The model under review builds one solid part; all positions refer to its coordinate system, in mm. A direction names the side the tool comes from. Round coordinates to 2 decimals unless told otherwise and drop trailing zeros. Order: outer loops, then holes, each group sorted by start corner. A loop starts at its lowest first (then second) coordinate and runs counter-clockwise, first axis right, second up.
1) Mouldability with a two-part tool opening along Z and no side actions: class faces 3 (the face through (38.1, 2, -3)), 4 (the face through (19, 1, 7.62)), 5 (the face through (34.148, 1.252, 1.164)) as pulls with the +Z half, pulls with the -Z half, needs draft (parallel to the pull), parting line crosses it, or undercut.
2) Consider section A-A (x = 31.75). Give the boundary of the cut face in (y, z).
3) To check wall thickness, follow L1, parallel to Z at x = 6.35, y = 1.75; L2, parallel to Y at x = 22.5, z = 0.75; L3, parallel to Z at x = 11, y = 7.5. State the ranges of each line that lie inside material, in increasing order.
4) Clearance check with flat-ended pins moving along their axes: P1, Ø2.5, axis at x = 27.5, y = 5.5, coming from the +Z side; P2, Ø3, axis at x = 4.5, y = 3.5, coming from the +Z side; P3, Ø7.5, axis at x = 22, z = -2, coming from the +Y side; P4, Ø3, axis at x = 31.75, z = 1.27, coming from the -Y side. State where each tip first meets the part, or that it passes through.
5) Machinability: for faces 1 (the face through (0, 2, -3)), 2 (the face through (19, 2.54, 0)), which of the approach directions +Z, -Z, +X, -X, +Y, -Y give a long, thin tool a straight path to every point of the face, cutting with its end or side? Answer none if there is none.
6) Consider section B-B (z = 1.27). Give the boundary of the cut face in (x, y).
7) Consider section C-C (y = 6.35). Give the boundary of the cut face in (x, z).
8) Consider section D-D (x = 3). Give the boundary of the cut face in (y, z).
from build123d import *

# Parameters (mm, degrees)
SKETCH2_W               = 10.16
SKETCH2_H               = 10.16
BOSS_EXTRUDE1_DEPTH     = 38.1
CUT_EXTRUDE1_DEPTH      = 41.719297636
CUT_EXTRUDE1_DEPTH_BACK = 38.1
SKETCH3_W               = 7.62
SKETCH3_H               = 7.62
M4_CLEARANCE_HOLE2_D    = 4.8
SKETCH13_W              = 38.1
SKETCH13_H              = 2.54
BOSS_EXTRUDE2_DEPTH     = 7.62
M4_CLEARANCE_HOLE3_D    = 4.8


with BuildPart() as part:
    # Sketch2 → Boss-Extrude1 (new body)
    with BuildSketch(Plane(origin=(0, 0, 0), x_dir=(0, 0, -1), z_dir=(1, 0, 0))):
        with Locations((5.08, 5.08)):
            Rectangle(SKETCH2_W, SKETCH2_H)
    extrude(amount=BOSS_EXTRUDE1_DEPTH)

    # Sketch3 → Cut-Extrude1 (cut, two sides: drawn at the far end of the back side and taken through both)
    with BuildSketch(Plane(origin=(38.1, 0, 0), x_dir=(0, 0, -1), z_dir=(1, 0, 0)).offset(-CUT_EXTRUDE1_DEPTH_BACK)):
        with Locations((3.81, 6.35)):
            Rectangle(SKETCH3_W, SKETCH3_H)
    extrude(amount=CUT_EXTRUDE1_DEPTH + CUT_EXTRUDE1_DEPTH_BACK, mode=Mode.SUBTRACT)

    # M4 Clearance Hole2 (through all)
    with Locations(Plane.XY.offset(-7.62)):
        with Locations((6.35, 6.35), (31.75, 6.35)):
            Hole(M4_CLEARANCE_HOLE2_D / 2)

    # Sketch13 → Boss-Extrude2 (add)
    with BuildSketch(Plane.XY):
        with Locations((19.05, 1.27)):
            Rectangle(SKETCH13_W, SKETCH13_H)
    extrude(amount=BOSS_EXTRUDE2_DEPTH)

    # M4 Clearance Hole3 (through all)
    with Locations(Plane(origin=(0, 2.54, 0), x_dir=(1, 0, 0), z_dir=(0, 1, 0))):
        with Locations((6.35, -1.27), (31.75, -1.27)):
            Hole(M4_CLEARANCE_HOLE3_D / 2)


solid = part.part
Answer below:
1. face 3: needs draft
1. face 4: pulls with the +Z half
1. face 5: undercut
2. outline: (0, -10.16) - (3.95, -10.16) - (3.95, -7.62) - (2.54, -7.62) - (2.54, -1.13) - (0, -1.13) - close; (0, 3.67) - (2.54, 3.67) - (2.54, 7.62) - (0, 7.62) - close; (8.75, -10.16) - (10.16, -10.16) - (10.16, -7.62) - (8.75, -7.62) - close
3. L1: z = -10.16 to -1.13, 3.67 to 7.62
3. L2: y = 0 to 2.54
3. L3: z = -10.16 to -7.62
4. P1: stops at z = -7.62
4. P2: stops at z = 7.62
4. P3: stops at y = 2.54
4. P4: passes through
5. face 1: +Z, -Z, -X, +Y, -Y
5. face 2: +Z, +X, -X, +Y
6. outline: (0, 0) - (3.95, 0) - (3.95, 2.54) - (0, 2.54) - close; (8.75, 0) - (29.35, 0) - (29.35, 2.54) - (8.75, 2.54) - close; (34.15, 0) - (38.1, 0) - (38.1, 2.54) - (34.15, 2.54) - close
7. outline: (0, -10.16) - (3.95, -10.16) - (3.95, -7.62) - (0, -7.62) - close; (8.75, -10.16) - (29.35, -10.16) - (29.35, -7.62) - (8.75, -7.62) - close; (34.15, -10.16) - (38.1, -10.16) - (38.1, -7.62) - (34.15, -7.62) - close
8. outline: (0, -10.16) - (10.16, -10.16) - (10.16, -7.62) - (2.54, -7.62) - (2.54, 7.62) - (0, 7.62) - close
